```python
from build123d import *

# Parameters (mm, degrees)
SKETCH3_W               = 76.2
SKETCH3_H               = 25.4
BOSS_EXTRUDE1_DEPTH     = 3.175
SKETCH4_W               = 38.1
SKETCH4_H               = 12.7
BOSS_EXTRUDE2_DEPTH     = 3.175
CUT_EXTRUDE1_DEPTH      = 38.1
CUT_EXTRUDE3_DEPTH      = 42.000549082
CUT_EXTRUDE3_DEPTH_BACK = 42.000549082
SKETCH12_W              = 1.5875
SKETCH12_H              = 10.16


with BuildPart() as part:
    # Sketch3 → Boss-Extrude1 (new body)
    with BuildSketch(Plane(origin=(0, 0, 0), x_dir=(1, 0, 0), z_dir=(0, 1, 0))):
        Rectangle(SKETCH3_W, SKETCH3_H)
    extrude(amount=BOSS_EXTRUDE1_DEPTH)

    # Sketch4 → Boss-Extrude2 (add)
    with BuildSketch(Plane(origin=(0, 3.175, 0), x_dir=(1, 0, 0), z_dir=(0, 1, 0))):
        with Locations((-19.05, 0)):
            Rectangle(SKETCH4_W, SKETCH4_H)
    extrude(amount=BOSS_EXTRUDE2_DEPTH)

    # Sketch6 → Cut-Extrude1 (cut)
    with BuildSketch(Plane.ZY.offset(38.1)):
        Polygon((-5.08, 1.905), (-5.08, 5.08), (-3.175, 5.08), (-3.175, 6.35), (3.175, 6.35), (3.175, 5.08), (5.08, 5.08), (5.08, 1.905), align=None)
    extrude(amount=-CUT_EXTRUDE1_DEPTH, mode=Mode.SUBTRACT)

    # Sketch11 → Revolve1 (revolve)
    with BuildSketch(Plane.XY, mode=Mode.PRIVATE) as revolve1_sk:
        Polygon((30.734, 3.175), (28.575, 3.175), (28.575, 6.731), (28.067, 7.493), (30.116415016, 8.255), (30.734, 8.255), align=None)
    revolve(revolve1_sk.sketch.rotate(Axis((31.75, 3.175, 0), (0, 1, 0)), 270), axis=Axis((31.75, 3.175, 0), (0, 1, 0)))

    # Sketch12 → Cut-Extrude3 (cut, two sides: drawn at the far end of the back side and taken through both)
    with BuildSketch(Plane.XY.offset(-CUT_EXTRUDE3_DEPTH_BACK)):
        with Locations((31.75, 8.255)):
            Rectangle(SKETCH12_W, SKETCH12_H)
    extrude(amount=CUT_EXTRUDE3_DEPTH + CUT_EXTRUDE3_DEPTH_BACK, mode=Mode.SUBTRACT)


solid = part.part
```
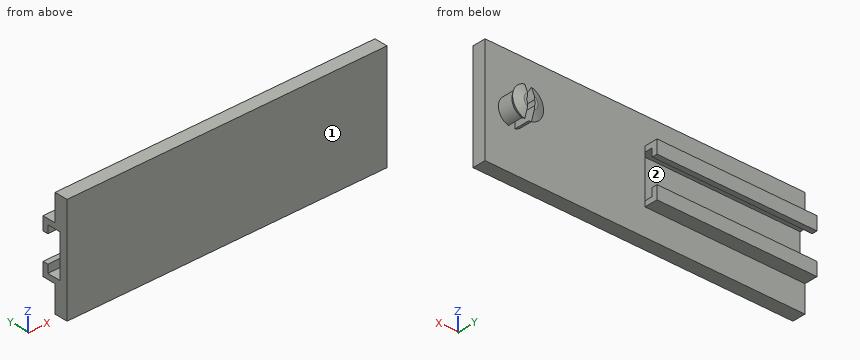
Part model, mm, in its own coordinate system. Face numbers are marked on the shaded views. Round coordinates to 2 decimals unless told otherwise and drop trailing zeros. Loops run counter-clockwise (first coordinate to the right, second up) from the corner with the lowest first, then second, coordinate; pieces in that order, holes last.
1. Slice it at C-C (x = 18). Give the cut face in (y, z) (3 decimals).
Solutions:
outline: (0, -12.7) - (3.175, -12.7) - (3.175, 12.7) - (0, 12.7) - close
2. Flat gauge pins, fed straight in: pin 1 (3.5 mm diameter, centred on x = -20.5, z = 5.5, fed in from +Y); pin 2 (3.5 mm diameter, centred on x = -15.5, y = 5.5, fed in from -Z); pin 3 (3.5 mm diameter, centred on x = -16, y = 5, fed in from +Z). Where does each tip first touch, or does it go through?
Solutions:
pin 1: stops at y = 6.35
pin 2: stops at z = -6.35
pin 3: stops at z = 6.35
3. Drill centre lines: line 1 along Z through (x, y) = (-2, 5.25) (3 decimals); line 2 along Y through (x, z) = (10.5, 7.5) (3 decimals); line 3 along X through (y, z) = (4.25, -5.75). Where is each one in solid material? Low to high.
Solutions:
line 1: z = -6.35 to -3.175, 3.175 to 6.35
line 2: y = 0 to 3.175
line 3: x = -38.1 to 0
4. Two-plate mould, pull along Z, no slides. Class the marked faces 1 and 2: pulls with the +Z half, pulls with the -Z half, needs draft (parallel to the pull), parting line crosses it, or undercut.
Solutions:
face 1: needs draft
face 2: undercut
5. Slice it at D-D (z = -10.25). Give the cut face in (x, y) (3 decimals).
Solutions:
outline: (-38.1, 0) - (38.1, 0) - (38.1, 3.175) - (-38.1, 3.175) - close
6. Slice it at A-A (z = -4.25). Give the cut face in (x, y) (3 decimals), and give its area (3 significant figures).
Solutions:
outline: (-38.1, 0) - (38.1, 0) - (38.1, 3.175) - (0, 3.175) - (0, 1.905) - (-38.1, 1.905) - close; (-38.1, 5.08) - (0, 5.08) - (0, 6.35) - (-38.1, 6.35) - close
area: 242 mm2
7. Slice it at B-B (y = 4). Give the cut face in (x, z) (3 decimals), and give its area (3 significant figures).
Solutions:
outline: (-38.1, -6.35) - (0, -6.35) - (0, -5.08) - (-38.1, -5.08) - close; (-38.1, 5.08) - (0, 5.08) - (0, 6.35) - (-38.1, 6.35) - close; (30.956, -3.074) - (30.956, -0.634) arc R1.016 cw to (30.956, 0.634) - (30.956, 3.074) arc R3.175 ccw to start; (32.544, -3.074) arc R3.175 ccw to (32.544, 3.074) - (32.544, 0.634) arc R1.016 cw to (32.544, -0.634) - close
area: 118 mm2
